```python
from build123d import *

# Parameters (mm, degrees)
BOSS_EXTRUDE1_DEPTH = 2.54
FILLET3_R           = 5.08
FILLET4_R           = 5.08
FILLET5_R           = 5.08
FILLET6_R           = 5.08
FILLET7_R           = 5.08
FILLET8_R           = 5.08
FILLET9_R           = 5.08
FILLET10_R          = 5.08


with BuildPart() as part:
    # Sketch2 → Boss-Extrude1 (new body)
    with BuildSketch(Plane(origin=(0, 0, 0), x_dir=(1, 0, 0), z_dir=(0, 1, 0))):
        with BuildLine():
            Line((-59.3725, 122.102714319), (-59.3725, 151.584711055))
            Line((-59.3725, 151.584711055), (59.3725, 151.584711055))
            Line((59.3725, 151.584711055), (59.3725, 122.102714319))
            ThreePointArc((59.3725, 122.102714319), (33.4645, 56.499868893), (59.3725, -9.102976533))
            Line((59.3725, -9.102976533), (59.3725, -51.615288945))
            Line((59.3725, -51.615288945), (-59.3725, -51.615288945))
            Line((-59.3725, -51.615288945), (-59.3725, -9.102976533))
            ThreePointArc((-59.3725, -9.102976533), (-33.4645, 56.499868893), (-59.3725, 122.102714319))
        make_face()
    extrude(amount=BOSS_EXTRUDE1_DEPTH)

    # Fillet3
    fillet3_edges = [part.edges().sort_by_distance(p)[0] for p in [
        (-59.3725, 1.27, -151.584711055),
    ]]
    fillet(fillet3_edges, radius=FILLET3_R)

    # Fillet4
    fillet4_edges = [part.edges().sort_by_distance(p)[0] for p in [
        (59.3725, 1.27, -151.584711055),
    ]]
    fillet(fillet4_edges, radius=FILLET4_R)

    # Fillet5
    fillet5_edges = [part.edges().sort_by_distance(p)[0] for p in [
        (-59.3725, 1.27, -122.102714319),
    ]]
    fillet(fillet5_edges, radius=FILLET5_R)

    # Fillet6
    fillet6_edges = [part.edges().sort_by_distance(p)[0] for p in [
        (59.3725, 1.27, -122.102714319),
    ]]
    fillet(fillet6_edges, radius=FILLET6_R)

    # Fillet7
    fillet7_edges = [part.edges().sort_by_distance(p)[0] for p in [
        (-59.3725, 1.27, 9.102976533),
    ]]
    fillet(fillet7_edges, radius=FILLET7_R)

    # Fillet8
    fillet8_edges = [part.edges().sort_by_distance(p)[0] for p in [
        (59.3725, 1.27, 9.102976533),
    ]]
    fillet(fillet8_edges, radius=FILLET8_R)

    # Fillet9
    fillet9_edges = [part.edges().sort_by_distance(p)[0] for p in [
        (59.3725, 1.27, 51.615288945),
    ]]
    fillet(fillet9_edges, radius=FILLET9_R)

    # Fillet10
    fillet10_edges = [part.edges().sort_by_distance(p)[0] for p in [
        (-59.3725, 1.27, 51.615288945),
    ]]
    fillet(fillet10_edges, radius=FILLET10_R)


solid = part.part
```
Can you work these out from the model? Positions are in its coordinate system, mm. Coordinates: 2 decimals unless noted, no trailing zeros. Loops run counter-clockwise (first coordinate to the right, second up) from the corner with the lowest first, then second, coordinate; pieces in that order, holes last. Notation, with made-up numbers: M 69.5,-12 L 85.5,-12 A21 ccw 85.5,26 Z; hole C 3,48.5 d2. An arc over 180 degrees is marked long. Put each result on its own line as item: value. Start each with the question number.
(1) Imagine slicing it at D-D on x = 40. List the corners of the cut face in (y, z) for me, and give its area (3 significant figures).
(2) Imagine slicing it at A-A on x = -45. List the corners of the cut face in (y, z) for me, and give its area (3 significant figures).
(3) Imagine slicing it at C-C on z = -104.5. List the corners of the cut face in (x, y) for me, and give its area (3 significant figures).
(4) Imagine slicing it at B-B on y = 0.8. List the corners of the cut face in (x, z) for me, and give its area (3 significant figures).
(5) We'd pull the mould along Z, two halves only. Please class faces 1 (the face through (-57.84, 1.29, 50.17)), 2 (the face through (-33.47, 1.25, -55.52)), 3 (the face through (1, 0, -51)): +Z half, -Z half, draft (parallel to the pull), parting line (faces both ways), or undercut.
(6) Will these pins go through, and if not, where does the flat tip stop? pin 1 Ø3 at (x, z) = (-31, 5) entering from -Y; pin 2 Ø2 at (x, z) = (-44, -16) entering from +Y.
(7) I need wall thicknesses on probe 1 along X at (y, z) = (0.8, -56.5); probe 2 along Z at (x, y) = (45, 0.9); probe 3 along Z at (x, y) = (47, 1.9). Which ranges of each line are inside material? Lowest first, please.
Worked answers:
1. outline: M 0,-151.58 L 2.54,-151.58 L 2.54,-91.32 L 0,-91.32 Z; M 0,-21.68 L 2.54,-21.68 L 2.54,51.62 L 0,51.62 Z
1. area: 339 mm2
2. outline: M 0,-151.58 L 2.54,-151.58 L 2.54,-102.13 L 0,-102.13 Z; M 0,-10.87 L 2.54,-10.87 L 2.54,51.62 L 0,51.62 Z
2. area: 284 mm2
3. outline: M -46.32,0 L 46.32,0 L 46.32,2.54 L -46.32,2.54 Z
3. area: 235 mm2
4. outline: M -59.37,-146.5 A5.08 ccw -54.29,-151.58 L 54.29,-151.58 A5.08 ccw 59.37,-146.5 L 59.37,-124.08 A5.08 ccw 58.07,-120.68 A96.01 cw 58.07,7.68 A5.08 ccw 59.37,11.08 L 59.37,46.54 A5.08 ccw 54.29,51.62 L -54.29,51.62 A5.08 ccw -59.37,46.54 L -59.37,11.08 A5.08 ccw -58.07,7.68 A96.01 cw -58.07,-120.68 A5.08 ccw -59.37,-124.08 Z
4. area: 19,400 mm2
5. face 1: +Z half
5. face 2: undercut
5. face 3: draft
6. pin 1: stops at y = 0
6. pin 2: passes through
7. probe 1: x = -33.46 to 33.46
7. probe 2: z = -151.58 to -102.13, -10.87 to 51.62
7. probe 3: z = -151.58 to -105.65, -7.35 to 51.62
